from build123d import *

# Parameters (mm, degrees)
SKETCH2_R           = 5
BOSS_EXTRUDE1_DEPTH = 50
SKETCH3_R           = 10.087575419
BOSS_EXTRUDE2_DEPTH = 12
CHAMFER1_SIZE       = 2
FILLET2_R           = 2
FILLET3_R           = 2


with BuildPart() as part:
    # Sketch2 → Boss-Extrude1 (new body)
    with BuildSketch(Plane(origin=(0, 0, 0), x_dir=(1, 0, 0), z_dir=(0, 1, 0))):
        with Locations(Location((0, 0, 0), (0, 0, 270))):
            Circle(SKETCH2_R)
    extrude(amount=BOSS_EXTRUDE1_DEPTH)

    # Sketch3 → Boss-Extrude2 (add)
    with BuildSketch(Plane.XZ):
        with Locations(Location((0, 0, 0), (0, 0, 270))):
            Circle(SKETCH3_R)
    extrude(amount=BOSS_EXTRUDE2_DEPTH)

    # Chamfer1
    chamfer1_edges = [part.edges().sort_by_distance(p)[0] for p in [
        (0, 0, 10.087575419),
    ]]
    chamfer(chamfer1_edges, length=CHAMFER1_SIZE)

    # Fillet2
    fillet2_edges = [part.edges().sort_by_distance(p)[0] for p in [
        (0, 0, 8.087575419),
    ]]
    fillet(fillet2_edges, radius=FILLET2_R)

    # Fillet3
    fillet3_edges = [part.edges().sort_by_distance(p)[0] for p in [
        (0, -2, 10.087575419),
    ]]
    fillet(fillet3_edges, radius=FILLET3_R)


solid = part.part
Could you check a few things on this model? Use its own coordinates, in mm. A direction names the side the tool comes from. Coordinates: 2 decimals unless noted, no trailing zeros. Loops run counter-clockwise (first coordinate to the right, second up) from the corner with the lowest first, then second, coordinate; pieces in that order, holes last. Notation, with made-up numbers: (-15, 81.25) -> (32, 81.25) arc R10 ccw to (32, 97.25) -> close; hole circle Ø5 at (18.5, 89.5). An arc over 180 degrees is marked (long way). Answer in a Markdown table with one row per item.
(1) Will these pins go through, and if not, where does the flat tip stop? pin 1 Ø4 at (x, y) = (6, 6) entering from -Z; pin 2 Ø10 at (y, z) = (19, 2.5) entering from -X; pin 3 Ø8 at (x, y) = (-6, 5.5) entering from +Z.
Results found:
| item | result |
|---|---|
| pin 1 | stops at z = -3 |
| pin 2 | stops at x = -5 |
| pin 3 | stops at z = 4.58 |
(2) Imagine slicing it at A-A (y = 41). List the corners of the cut face in (x, z) for me, plus the area to 3 significant figures.
Results found:
| item | result |
|---|---|
| outline | circle Ø10 at (0, 0) |
| area | 78.5 mm^2 |
(3) For faces 1 (the face through (2, 0, -5)), 2 (the face through (0, 50, 0)), which set-ups out of +Z, -Z, +X, -X, +Y, -Y let a thin tool reach every point of the face, with its end or its side?
Results found:
| item | result |
|---|---|
| face 1 | +Y |
| face 2 | +Z, -Z, +X, -X, +Y |
(4) If I drill on probe 1 along X at (y, z) = (24, -0.25); probe 2 along Y at (x, z) = (-9, -3); probe 3 along Y at (x, z) = (6.75, -2.25), over which ranges is the centre line in solid material (lowest first)?
Results found:
| item | result |
|---|---|
| probe 1 | x = -4.99 to 4.99 |
| probe 2 | y = -12 to -1.4 |
| probe 3 | y = -12 to 0 |
